```python
from build123d import *

# Parameters (mm, degrees)
EXTRUDE_1_DEPTH   = 2
HOLE_WIZARD_M81_D = 9
CHAMFER_1_SIZE    = 2


with BuildPart() as part:
    # Эскиз1 → Бобышка-Вытянуть1 (new body)
    with BuildSketch(Plane(origin=(0, 0, 0), x_dir=(1, 0, 0), z_dir=(0, 0, -1))):
        Polygon((-45, 135), (45, 135), (45, 90), (22.5, 90), (22.5, 0), (-22.5, 0), (-22.5, 90), (-45, 90), align=None)
    extrude(amount=EXTRUDE_1_DEPTH)

    # Отверстие с зазором M81 (through all)
    with Locations(Plane(origin=(0, 0, -2), x_dir=(1, 0, 0), z_dir=(0, 0, -1))):
        with Locations((0, 22.5), (-22.5, 112.5), (22.5, 112.5), (0, 67.5)):
            Hole(HOLE_WIZARD_M81_D / 2)

    # Фаска1
    chamfer_1_edges = [part.edges().sort_by_distance(p)[0] for p in [
        (-45, -90, -1),
        (-45, -135, -1),
        (45, -135, -1),
        (45, -90, -1),
        (22.5, 0, -1),
        (-22.5, 0, -1),
    ]]
    chamfer(chamfer_1_edges, length=CHAMFER_1_SIZE)


solid = part.part
```
Input: part model. Units: mm. Frame: model coordinates. Coordinates: 2 decimals unless noted, no trailing zeros. Loops run counter-clockwise (first coordinate to the right, second up) from the corner with the lowest first, then second, coordinate; pieces in that order, holes last.
Q1. Section A-A, the plane y = -67.5. Return the cut outline in (x, z), and give its area (3 significant figures).
Results are:
outline: (-22.5, -2) - (-4.5, -2) - (-4.5, 0) - (-22.5, 0) - close; (4.5, -2) - (22.5, -2) - (22.5, 0) - (4.5, 0) - close
area: 72.0 mm2
Q2. Line query: line 1 along X through (y, z) = (-112.5, -1.3); line 2 along Y through (x, z) = (0, -0.95); line 3 along X through (y, z) = (-22.5, -0.4). Output: solid intervals per line, ascending.
Results are:
line 1: x = -45 to -27, -18 to 18, 27 to 45
line 2: y = -135 to -72, -63 to -27, -18 to 0
line 3: x = -22.5 to -4.5, 4.5 to 22.5
Q3. Section D-D, the plane x = 0. Return the cut outline in (y, z).
Results are:
outline: (-135, -2) - (-72, -2) - (-72, 0) - (-135, 0) - close; (-63, -2) - (-27, -2) - (-27, 0) - (-63, 0) - close; (-18, -2) - (0, -2) - (0, 0) - (-18, 0) - close
Q4. Contact query for a flat-ended pin moving along its axis: pin 1 (0.6 mm diameter, centred on x = 34, z = -0.5, fed in from +Y). Output: stop coordinate, or through.
Results are:
pin 1: stops at y = -90
Q5. Mould query, pull axis X, two halves, no side actions, for faces 1 (the flat face through (1, -83, 0)), 2 (the cylindrical face through (23.09, -116.96, -0.99)). Classes: +X half, -X half, draft (parallel to the pull), parting line (faces both ways), or undercut.
Results are:
face 1: draft
face 2: undercut
Q6. Section B-B, the plane z = -0.5. Return the cut outline in (x, y).
Results are:
outline: (-45, -133) - (-43, -135) - (43, -135) - (45, -133) - (45, -92) - (43, -90) - (22.5, -90) - (22.5, -2) - (20.5, 0) - (-20.5, 0) - (-22.5, -2) - (-22.5, -90) - (-43, -90) - (-45, -92) - close; hole circle Ø9 at (-22.5, -112.5); hole circle Ø9 at (0, -67.5); hole circle Ø9 at (0, -22.5); hole circle Ø9 at (22.5, -112.5)
Q7. Section C-C, the plane y = -112.5. Return the cut outline in (x, z), and give its area (3 significant figures).
Results are:
outline: (-45, -2) - (-27, -2) - (-27, 0) - (-45, 0) - close; (-18, -2) - (18, -2) - (18, 0) - (-18, 0) - close; (27, -2) - (45, -2) - (45, 0) - (27, 0) - close
area: 144 mm2
